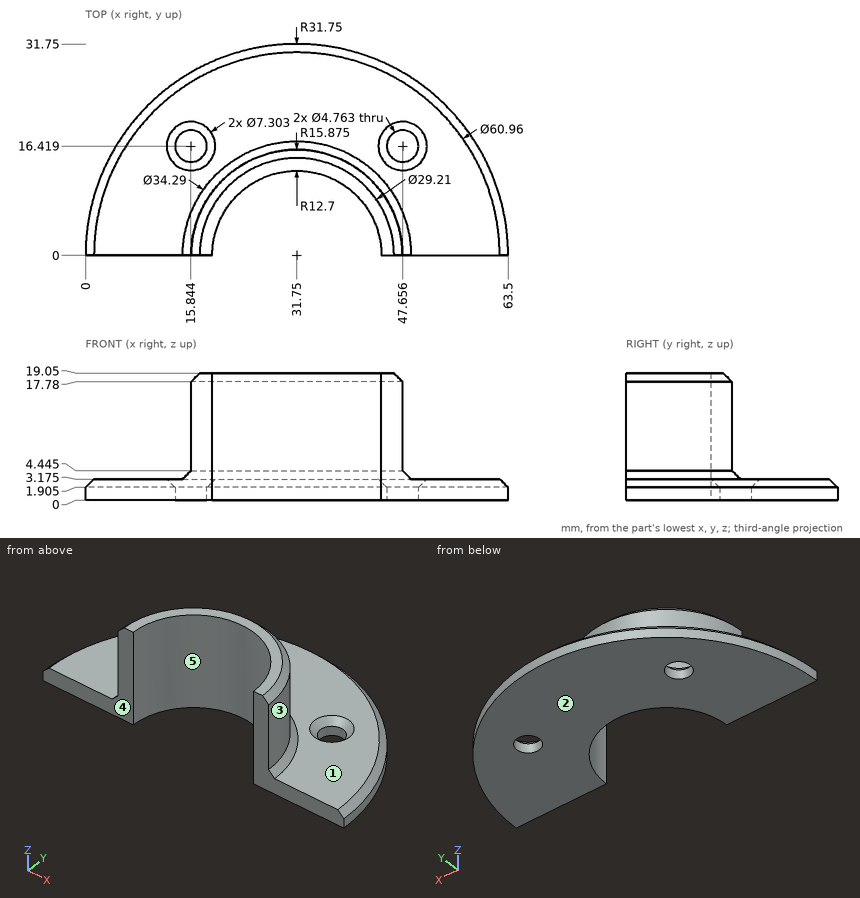
The drawing under review shows one solid part. Ordinate dimensions are in mm from its lowest x, y, z. A direction names the side the tool comes from. Coordinates: 2 decimals unless noted, no trailing zeros.
Item 1: Draft analysis for pull direction X (two halves, no side actions). For the marked faces 3, 4 and 5, state which applies: pulls with the +X half, pulls with the -X half, needs draft (parallel to the pull), parting line crosses it, or undercut.
Completed:
face 3: parting line crosses it
face 4: needs draft
face 5: undercut
Item 2: Clearance check with flat-ended pins moving along their axes: pin 1 (6 mm diameter, centred on y = 4.5, z = 14.5, fed in from -X); pin 2 (5 mm diameter, centred on x = 41, y = 23.5, fed in from +Z) (1 decimal); pin 3 (4 mm diameter, centred on x = 28.5, z = 7.5, fed in from +Y). State where each tip first meets the part, or that it passes through.
Completed:
pin 1: stops at x = 15.95
pin 2: stops at z = 3.2
pin 3: stops at y = 15.83
Item 3: Wall thickness on L1, parallel to Z at x = 60, y = 10.5 (1 decimal); L2, parallel to Y at x = 31.5, z = 11.5; L3, parallel to X at y = 5, z = 7 (1 decimal): over which ranges is each line inside the solid? List them lowest first.
Completed:
L1: z = 0 to 3.2
L2: y = 12.7 to 15.87
L3: x = 16.7 to 20.1, 43.4 to 46.8
Item 4: For the marked faces 1 and 2, list the 3-axis set-ups (+Z, -Z, +X, -X, +Y, -Y) from which the entire face can be reached by the end or side of a thin tool; tool diameter is ignored.
Completed:
face 1: +Z, +Y
face 2: -Z, +X, -X, +Y, -Y
